Could you check a few things on this model? Use its own coordinates, in mm. A direction names the side the tool comes from. Coordinates: 2 decimals unless noted, no trailing zeros. Write each loop counter-clockwise with the first axis right and the second up, starting at its lowest first coordinate (ties: lowest second). Pieces come first, ordered by that corner, then holes. Notation, with made-up numbers: (-37, -3) - (12, -3) arc R23 ccw to (12, 16) - close; hole circle Ø8 at (75, 76). An arc over 180 degrees is marked (long way). Answer as a JSON object with one key per item and string values. Group by question number.
1) If we section it at D-D (y = 50.5): Write out the boundary of the cut face in (x, z).
2) On a 3-axis mill with a long thin cutter (end or side, diameter ignored), from which of +Z, -Z, +X, -X, +Y, -Y can I reach the whole of each face in a straight line? I mean faces 1 (the flat face through (17.4, 5, 4.9)), 2 (the flat face through (0, 48, 5)). Say none if no direction works.
3) If we section it at C-C (z = 9): Write out the boundary of the cut face in (x, y).
4) If we section it at B-B (x = 14.75): Write out the boundary of the cut face in (y, z).
5) Will these pins go through, and if not, where does the flat tip stop? pin 1 Ø2 at (x, y) = (3.5, 68.5) entering from -Z; pin 2 Ø3 at (x, z) = (12.5, 5) entering from +Y; pin 3 Ø1.5 at (y, z) = (69, 3) entering from +X.
6) If we section it at A-A (z = 5): Write out the boundary of the cut face in (x, y).
7) We'd pull the mould along Z, two halves only. Please class faces 3 (the flat face through (5, 49, 5)), 4 (the cylindrical face through (13, 2, 5)), 5 (the flat face through (4, 41, 0)): released by +Z, released by -Z, zero draft, split by the parting line, or undercut.
8) Please list where these lines run through material, in increasing order: line 1 along Z through (x, y) = (15, 1); line 2 along Y through (x, z) = (12.75, 9.5).
```python
from build123d import *

# Parameters (mm, degrees)
PAD_DEPTH   = 10
SKETCH001_R = 2
HOLE_DEPTH  = 23.798279
HOLE_TIPS_R = 2


with BuildPart() as part:
    # Sketch → Pad (new body)
    with BuildSketch(Plane.XY):
        Polygon((0, 95), (0, 0), (25, 0), (25, 5), (5, 5), (5, 95), align=None)
    extrude(amount=PAD_DEPTH)

    # Sketch001 (on Face2 of Pad) → Hole (cut)
    with BuildSketch(Plane.XZ):
        with Locations((15, 5)):
            Circle(SKETCH001_R)
    extrude(amount=-HOLE_DEPTH, mode=Mode.SUBTRACT)

    # Hole tips → Hole tip 1 section 0
    with BuildSketch(Plane.XZ.offset(-23.798279), mode=Mode.PRIVATE) as hole_tip_1_s0:
        with Locations((15, 5)):
            Circle(HOLE_TIPS_R)
    loft([hole_tip_1_s0.sketch, Vertex(15, 25, 5)], mode=Mode.SUBTRACT)


solid = part.part
```
Here are the results:
{
 "1": {"outline": "(0, 0) - (5, 0) - (5, 10) - (0, 10) - close"},
 "2": {"face 1": "+Z, -Z, +X, +Y", "face 2": "+Z, -Z, -X, +Y, -Y"},
 "3": {"outline": "(0, 0) - (25, 0) - (25, 5) - (5, 5) - (5, 95) - (0, 95) - close"},
 "4": {"outline": "(0, 0) - (5, 0) - (5, 3.02) - (0, 3.02) - close; (0, 6.98) - (5, 6.98) - (5, 10) - (0, 10) - close"},
 "5": {"pin 1": "stops at z = 0", "pin 2": "stops at y = 5", "pin 3": "stops at x = 5"},
 "6": {"outline": "(0, 0) - (13, 0) - (13, 5) - (5, 5) - (5, 95) - (0, 95) - close; (17, 0) - (25, 0) - (25, 5) - (17, 5) - close"},
 "7": {"face 3": "zero draft", "face 4": "undercut", "face 5": "released by -Z"},
 "8": {"line 1": "z = 0 to 3, 7 to 10", "line 2": "y = 0 to 5"}
}
